Model file for the job. Use its own axes, mm. A direction names the side the tool comes from. Round coordinates to 2 decimals unless told otherwise and drop trailing zeros. Loops run counter-clockwise (first coordinate to the right, second up) from the corner with the lowest first, then second, coordinate; pieces in that order, holes last. Notation, with made-up numbers: (58, -35) -> (109, -35) arc R28 ccw to (109, -7) -> close; hole circle Ø8 at (-13.75, -17.5). An arc over 180 degrees is marked (long way). Use a Markdown table: item, result. Add a question column.
```python
from build123d import *

# Parameters (mm, degrees)
F0_R     = 36
F0_R_2   = 30
F1_DEPTH = 13
F0_R_3   = 50
F0_R_4   = 2.1
F2_DEPTH = 30
F3_DEPTH = 13


with BuildPart() as f1:
    # F0 (on Front) → F1 (new body)
    with BuildSketch(Plane.XZ):
        with Locations((-81.370543, 0)):
            Circle(F0_R)
        with Locations((-81.370543, 0)):
            Circle(F0_R_2, mode=Mode.SUBTRACT)
    extrude(amount=F1_DEPTH)

    # F0 (on Front) → F2 (join)
    with BuildSketch(Plane.XZ):
        with Locations((-81.370543, 0)):
            Circle(F0_R_3)
        with Locations((-123.541678, -18.964189)):
            Circle(F0_R_4, mode=Mode.SUBTRACT)
        with Locations((-38.513874, -17.330143)):
            Circle(F0_R_4, mode=Mode.SUBTRACT)
        with Locations((-82.265135, 46.239)):
            Circle(F0_R_4, mode=Mode.SUBTRACT)
        with Locations((-81.370543, 0)):
            Circle(F0_R, mode=Mode.SUBTRACT)
    extrude(amount=F2_DEPTH)

    # F0 (on Front) → F3 (join)
    with BuildSketch(Plane.XZ):
        with Locations((-123.541678, -18.964189)):
            Circle(F0_R_4)
        with Locations((-82.265135, 46.239)):
            Circle(F0_R_4)
        with Locations((-38.513874, -17.330143)):
            Circle(F0_R_4)
    extrude(amount=F3_DEPTH)


solid = f1.part
```
1) Cut at A-A on z = 0. Write the cut outline in (x, y).
2) Cut at B-B on x = -107. Write the cut outline in (y, z).
3) Cut at D-D on y = -24.75. Write the cut outline in (x, z), and give its area (3 significant figures).
4) Pin check, flat tips, straight feed: pin 1 Ø12 at (y, z) = (-8, -34) entering from -X; pin 2 Ø4 at (x, y) = (-94.5, -3) entering from +Z; pin 3 Ø2 at (x, y) = (-61.5, -23.5) entering from +Z. Stop position of each tip, or through.
5) Cut at C-C on y = -4.5. Write the cut outline in (x, z).
6) Pull direction Z, two halves, no side cores. Call faces 1 (the face through (-121.05, -14.79, -30.42)), 2 (the face through (-66.8, -30, -33.1)), 3 (the face through (-39, -13, -17)): +Z half, -Z half, draft (parallel to the pull), parting line (faces both ways), or undercut.
7) Tool access for faces 4 (the face through (-47.03, -21.38, 10.81)), 5 (the face through (-111.34, -6.41, 1.32)): list every direction of +Z, -Z, +X, -X, +Y, -Y with a clear straight run to the whole face (end or side of a thin tool).
8) Wall check: probe 1 along X at (y, z) = (-6, -18.5); probe 2 along Z at (x, y) = (-92, -2.5); probe 3 along Z at (x, y) = (-83.5, -6.5). Give the ranges that are in metal, low to high. Write a range as from..to.
Established:
| question | item | result |
|---|---|---|
| 1 | outline | (-131.37, -30) -> (-117.37, -30) -> (-117.37, -13) -> (-111.37, -13) -> (-111.37, 0) -> (-131.37, 0) -> close; (-51.37, -13) -> (-45.37, -13) -> (-45.37, -30) -> (-31.37, -30) -> (-31.37, 0) -> (-51.37, 0) -> close |
| 2 | outline | (-30, -42.93) -> (0, -42.93) -> (0, -15.59) -> (-13, -15.59) -> (-13, -25.28) -> (-30, -25.28) -> close; (-30, 25.28) -> (-13, 25.28) -> (-13, 15.59) -> (0, 15.59) -> (0, 42.93) -> (-30, 42.93) -> close |
| 3 | outline | circle Ø100 at (-81.37, 0); hole circle Ø4.2 at (-123.54, -18.96); hole circle Ø72 at (-81.37, 0); hole circle Ø4.2 at (-82.27, 46.24); hole circle Ø4.2 at (-38.51, -17.33) |
| 3 | area | 3,740 mm^2 |
| 4 | pin 1 | stops at x = -122.8 |
| 4 | pin 2 | stops at z = 48.75 |
| 4 | pin 3 | stops at z = 46.3 |
| 5 | outline | circle Ø100 at (-81.37, 0); hole circle Ø60 at (-81.37, 0) |
| 6 | face 1 | parting line |
| 6 | face 2 | draft |
| 6 | face 3 | undercut |
| 7 | face 4 | -Y |
| 7 | face 5 | +Y, -Y |
| 8 | probe 1 | x = -127.82..-104.99, -57.75..-34.92 |
| 8 | probe 2 | z = -48.86..-28.05, 28.05..48.86 |
| 8 | probe 3 | z = -49.95..-29.92, 29.92..49.95 |
